```python
from build123d import *

# Parameters (mm, degrees)
SKETCH2_W           = 26
SKETCH2_H           = 16
BOSS_EXTRUDE1_DEPTH = 2
SKETCH3_W           = 26
SKETCH3_H           = 16
SKETCH3_W_2         = 22.5
SKETCH3_H_2         = 13
BOSS_EXTRUDE2_DEPTH = 22
CUT_EXTRUDE1_REACH  = 40.833
CUT_EXTRUDE2_REACH  = 40.833
CUT_EXTRUDE3_REACH  = 40.833
CUT_EXTRUDE4_REACH  = 40.833
SKETCH10_R          = 2.3
BOSS_EXTRUDE3_DEPTH = 8.56
BOSS_EXTRUDE4_START = 8.56
SKETCH11_R          = 2.3
BOSS_EXTRUDE4_DEPTH = 8.56
SKETCH12_R          = 1.65
CUT_EXTRUDE5_DEPTH  = 8.56
CUT_EXTRUDE6_START  = -8.56
SKETCH13_R          = 1.65
CUT_EXTRUDE6_DEPTH  = 8.56


with BuildPart() as part:
    # Sketch2 → Boss-Extrude1 (new body)
    with BuildSketch(Plane(origin=(0, 0, 0), x_dir=(1, 0, 0), z_dir=(0, 1, 0))):
        with Locations((13, 8)):
            Rectangle(SKETCH2_W, SKETCH2_H)
    extrude(amount=BOSS_EXTRUDE1_DEPTH)

    # Sketch3 → Boss-Extrude2 (add)
    with BuildSketch(Plane(origin=(0, 2, 0), x_dir=(1, 0, 0), z_dir=(0, 1, 0))):
        with Locations((13, 8)):
            Rectangle(SKETCH3_W, SKETCH3_H)
        with Locations((13, 8)):
            Rectangle(SKETCH3_W_2, SKETCH3_H_2, mode=Mode.SUBTRACT)
    extrude(amount=BOSS_EXTRUDE2_DEPTH)

    # Sketch6 → Cut-Extrude1 (cut, up to next)
    with BuildSketch(Plane.ZY, mode=Mode.PRIVATE) as cut_extrude1_sk1:
        Polygon((-14.5, 24), (-14.5, 15), (-10, 15), (-10, 4), (-6, 4), (-6, 15), (-1.5, 15), (-1.5, 24), align=None)
    cut_extrude1_tool1 = extrude(cut_extrude1_sk1.sketch, amount=-CUT_EXTRUDE1_REACH, mode=Mode.PRIVATE) & part.part
    add(cut_extrude1_tool1.solids().sort_by_distance((0, 16.767081, -8))[0], mode=Mode.SUBTRACT)

    # Sketch7 → Cut-Extrude2 (cut, up to next)
    with BuildSketch(Plane(origin=(26, 0, 0), x_dir=(0, 0, -1), z_dir=(1, 0, 0)), mode=Mode.PRIVATE) as cut_extrude2_sk1:
        Polygon((1.5, 24), (1.5, 15), (6, 15), (6, 4), (10, 4), (10, 15), (14.5, 15), (14.5, 24), align=None)
    cut_extrude2_tool1 = extrude(cut_extrude2_sk1.sketch, amount=-CUT_EXTRUDE2_REACH, mode=Mode.PRIVATE) & part.part
    add(cut_extrude2_tool1.solids().sort_by_distance((26, 16.767081, -8))[0], mode=Mode.SUBTRACT)

    # Sketch8 → Cut-Extrude3 (cut, up to next)
    with BuildSketch(Plane(origin=(0, 0, -16), x_dir=(-1, 0, 0), z_dir=(0, 0, -1)), mode=Mode.PRIVATE) as cut_extrude3_sk1:
        with BuildLine():
            Line((-24, 12), (-24, 9))
            ThreePointArc((-24, 9), (-22.535533906, 5.464466094), (-19, 4))
            Line((-19, 4), (-7, 4))
            ThreePointArc((-7, 4), (-3.464466094, 5.464466094), (-2, 9))
            Line((-2, 9), (-2, 12))
            ThreePointArc((-2, 12), (-3.464466094, 15.535533906), (-7, 17))
            Line((-7, 17), (-19, 17))
            ThreePointArc((-19, 17), (-22.535533906, 15.535533906), (-24, 12))
        make_face()
    cut_extrude3_tool1 = extrude(cut_extrude3_sk1.sketch, amount=-CUT_EXTRUDE3_REACH, mode=Mode.PRIVATE) & part.part
    add(cut_extrude3_tool1.solids().sort_by_distance((13, 10.5, -16))[0], mode=Mode.SUBTRACT)

    # Sketch9 → Cut-Extrude4 (cut, up to next)
    with BuildSketch(Plane.XY, mode=Mode.PRIVATE) as cut_extrude4_sk1:
        with BuildLine():
            Line((2, 12), (2, 9))
            ThreePointArc((2, 9), (3.464466094, 5.464466094), (7, 4))
            Line((7, 4), (19, 4))
            ThreePointArc((19, 4), (22.535533906, 5.464466094), (24, 9))
            Line((24, 9), (24, 12))
            ThreePointArc((24, 12), (22.535533906, 15.535533906), (19, 17))
            Line((19, 17), (7, 17))
            ThreePointArc((7, 17), (3.464466094, 15.535533906), (2, 12))
        make_face()
    cut_extrude4_tool1 = extrude(cut_extrude4_sk1.sketch, amount=-CUT_EXTRUDE4_REACH, mode=Mode.PRIVATE) & part.part
    add(cut_extrude4_tool1.solids().sort_by_distance((13, 10.5, 0))[0], mode=Mode.SUBTRACT)

    # Sketch10 → Boss-Extrude3 (add)
    with BuildSketch(Plane(origin=(0, 0, -16), x_dir=(-1, 0, 0), z_dir=(0, 0, -1))):
        with Locations(Location((-20.97, 20, 0), (0, 0, 180))):
            Circle(SKETCH10_R)
        with Locations(Location((-5.03, 20, 0), (0, 0, 180))):
            Circle(SKETCH10_R)
    extrude(amount=BOSS_EXTRUDE3_DEPTH)

    # Sketch11 → Boss-Extrude4 (add)
    with BuildSketch(Plane.XY.offset(BOSS_EXTRUDE4_START)):
        with Locations((5.03, 20)):
            Circle(SKETCH11_R)
        with Locations((20.97, 20)):
            Circle(SKETCH11_R)
    extrude(amount=-BOSS_EXTRUDE4_DEPTH)

    # Sketch12 → Cut-Extrude5 (cut)
    with BuildSketch(Plane(origin=(0, 0, -24.56), x_dir=(-1, 0, 0), z_dir=(0, 0, -1))):
        with Locations((-20.97, 20)):
            Circle(SKETCH12_R)
        with Locations((-5.03, 20)):
            Circle(SKETCH12_R)
    extrude(amount=-CUT_EXTRUDE5_DEPTH, mode=Mode.SUBTRACT)

    # Sketch13 → Cut-Extrude6 (cut)
    with BuildSketch(Plane.XY.offset(8.56).offset(CUT_EXTRUDE6_START)):
        with Locations(Location((5.03, 20, 0), (0, 0, 180))):
            Circle(SKETCH13_R)
        with Locations(Location((20.97, 20, 0), (0, 0, 180))):
            Circle(SKETCH13_R)
    extrude(amount=CUT_EXTRUDE6_DEPTH, mode=Mode.SUBTRACT)


solid = part.part
```
Check sheet for the modelled part. Datum: model origin and axes. Units: mm. A direction names the side the tool comes from. Give positions to 0.01 mm unless a question says otherwise; leave off trailing zeros. Order: outer loops, then holes, each group sorted by start corner. A loop starts at its lowest first (then second) coordinate and runs counter-clockwise, first axis right, second up. Notation, with made-up numbers: M 86.25,22 L 99.25,22 A25 ccw 99.25,40 Z; hole C 8,27.25 d1. An arc over 180 degrees is marked long. Answer in a Markdown table with one row per item. Add a question column.
Q1. Sectioned sample at D-D, the plane y = 14.25. Record the boundary of the cut face in (x, z).
Q2. Release check for a two-part mould opening along X. For faces 1 (the flat face through (5, 20, 0)), 2 (the flat face through (25, 10, -6)) record: released by +X, released by -X, zero draft, split by the parting line, or undercut.
Q3. Gauge pin test, flat ends, axial feed: pin 1 Ø2.5 at (x, y) = (5.03, 20) entering from +Z; pin 2 Ø0.9 at (x, y) = (25, 9) entering from -Z; pin 3 Ø6.5 at (x, z) = (8.5, -9) entering from +Y. Record the tip position at first contact, or that the pin passes through.
Q4. Sectioned sample at C-C, the plane z = -8.5. Record the boundary of the cut face in (x, y).
Q5. Thickness scan on L1, parallel to X at y = 10.75, z = -0.5; L2, parallel to Z at x = 5.5, y = 18.75; L3, parallel to Y at x = 5.03, z = 4. Record the ranges inside material, lowest first.
Q6. Sectioned sample at A-A, the plane z = -15. Record the boundary of the cut face in (x, y), and give its area (3 significant figures).
Q7. Sectioned sample at B-B, the plane x = 16.25. Record the boundary of the cut face in (y, z), and give its area (3 significant figures).
Q8. Access from +Z, -Z, +X, -X, +Y, -Y to the whole of each face (thin tool, end or side, straight path). Record for faces 3 (the flat face through (1, 15, -12)), 4 (the cylindrical face through (4, 5, -15)), 5 (the cylindrical face through (4.14, 21.39, -20.34)), 6 (the flat face through (1.75, 8, -5)).
Verdict:
| question | item | result |
|---|---|---|
| 1 | outline | M 0,-16 L 2.53,-16 L 2.53,-14.5 L 1.75,-14.5 L 1.75,-10 L 0,-10 Z; M 0,-6 L 1.75,-6 L 1.75,-1.5 L 2.53,-1.5 L 2.53,0 L 0,0 Z; M 23.47,-16 L 26,-16 L 26,-10 L 24.25,-10 L 24.25,-14.5 L 23.47,-14.5 Z; M 23.47,-1.5 L 24.25,-1.5 L 24.25,-6 L 26,-6 L 26,0 L 23.47,0 Z |
| 2 | face 1 | undercut |
| 2 | face 2 | zero draft |
| 3 | pin 1 | z = 0 |
| 3 | pin 2 | z = -16 |
| 3 | pin 3 | y = 2 |
| 4 | outline | M 0,0 L 26,0 L 26,4 L 24.25,4 L 24.25,2 L 1.75,2 L 1.75,4 L 0,4 Z |
| 5 | L1 | 0 to 2, 24 to 26 |
| 5 | L2 | -16 to -14.5, -1.5 to 0 |
| 5 | L3 | 17.7 to 18.35, 21.65 to 22.3 |
| 6 | outline | M 0,0 L 26,0 L 26,24 L 0,24 Z; hole M 2,9 A5 ccw 7,4 L 19,4 A5 ccw 24,9 L 24,12 A5 ccw 19,17 L 7,17 A5 ccw 2,12 Z |
| 6 | area | 359 mm² |
| 7 | outline | M 0,-16 L 4,-16 L 4,-14.5 L 2,-14.5 L 2,-1.5 L 4,-1.5 L 4,0 L 0,0 Z; M 17,-16 L 24,-16 L 24,-14.5 L 17,-14.5 Z; M 17,-1.5 L 24,-1.5 L 24,0 L 17,0 Z |
| 7 | area | 59.0 mm² |
| 8 | face 3 | +X, -X, +Y |
| 8 | face 4 | +Z, -Z |
| 8 | face 5 | -Z |
| 8 | face 6 | +Y |
